Build history of the part. All positions in model axes, mm. Give positions to 0.01 mm unless a question says otherwise; leave off trailing zeros. Order: outer loops, then holes, each group sorted by start corner. A loop starts at its lowest first (then second) coordinate and runs counter-clockwise, first axis right, second up. Notation, with made-up numbers: (79.25, 54.25) - (131.25, 54.25) arc R20 cw to (131.25, 73.25) - close; hole circle Ø4 at (40.25, -10). An arc over 180 degrees is marked (long way). Answer in a Markdown table with one row per item.
```python
from build123d import *

# Parameters (mm, degrees)
F1_DEPTH = 7.5
F3_DEPTH = 25
F5_DEPTH = 25
F6_W     = 60
F6_H     = 10
F7_DEPTH = 25
F8_R     = 10


with BuildPart() as f1:
    # F0 (on Front) → F1 (new body)
    with BuildSketch(Plane.XZ):
        with BuildLine():
            Line((-64.5, -10), (-64.5, 10))
            Line((-64.5, 10), (-36.2157287525, 10))
            ThreePointArc((-36.2157287525, 10), (-94.5, 0), (-36.2157287525, -10))
            Line((-36.2157287525, -10), (-64.5, -10))
        make_face()
        with BuildLine():
            Line((-36.2157287525, 10), (-64.5, 10))
            Line((-64.5, 10), (-64.5, -10))
            Line((-64.5, -10), (-36.2157287525, -10))
            ThreePointArc((-36.2157287525, -10), (-34.9320432104, -5.0730593618), (-34.5, 0))
            ThreePointArc((-34.5, 0), (-34.9320432104, 5.0730593618), (-36.2157287525, 10))
        make_face()
        with BuildLine():
            Line((47.1794919243, 10), (-36.2157287525, 10))
            ThreePointArc((-36.2157287525, 10), (-34.9320432104, 5.0730593618), (-34.5, 0))
            ThreePointArc((-34.5, 0), (-34.9320432104, -5.0730593618), (-36.2157287525, -10))
            Line((-36.2157287525, -10), (47.1794919243, -10))
            ThreePointArc((47.1794919243, -10), (44.5, 0), (47.1794919243, 10))
        make_face()
        with BuildLine():
            ThreePointArc((84.5, 0), (69.6763809021, 19.3185165258), (47.1794919243, 10))
            Line((47.1794919243, 10), (64.5, 10))
            Line((64.5, 10), (64.5, -10))
            Line((64.5, -10), (47.1794919243, -10))
            ThreePointArc((47.1794919243, -10), (69.6763809021, -19.3185165258), (84.5, 0))
        make_face()
        with BuildLine():
            Line((64.5, 10), (47.1794919243, 10))
            ThreePointArc((47.1794919243, 10), (44.5, 0), (47.1794919243, -10))
            Line((47.1794919243, -10), (64.5, -10))
            Line((64.5, -10), (64.5, 10))
        make_face()
    extrude(amount=F1_DEPTH)

    # F2 (on face) → F3 (cut)
    with BuildSketch(Plane.XZ.offset(7.5)):
        Polygon((-52.9529946162, 20), (-76.0470053838, 20), (-87.5940107676, 0), (-76.0470053838, -20), (-52.9529946162, -20), (-41.4059892324, 0), align=None)
    extrude(amount=-F3_DEPTH, mode=Mode.SUBTRACT)

    # F4 (on face) → F5 (cut)
    with BuildSketch(Plane.XZ.offset(7.5)):
        Polygon((73.3167787844, -12.1352549156), (78.7658477444, 4.6352549156), (64.5, 15), (50.2341522556, 4.6352549156), (55.6832212156, -12.1352549156), align=None)
    extrude(amount=-F5_DEPTH, mode=Mode.SUBTRACT)

    # F6 (on face) → F7 (cut)
    with BuildSketch(Plane.XZ.offset(7.5)):
        with Locations((6.0453672857, 0)):
            Rectangle(F6_W, F6_H)
        with BuildLine():
            ThreePointArc((-23.9546327143, 5), (-28.9546327143, 0), (-23.9546327143, -5))
            Line((-23.9546327143, -5), (-23.9546327143, 5))
        make_face()
        with BuildLine():
            Line((36.0453672857, 5), (36.0453672857, -5))
            ThreePointArc((36.0453672857, -5), (41.0453672857, 0), (36.0453672857, 5))
        make_face()
    extrude(amount=-F7_DEPTH, mode=Mode.SUBTRACT)

    # F8
    f8_edges = [f1.edges().sort_by_distance(p)[0] for p in [
        (-36.215729, -3.75, -10),
        (47.179492, -3.75, 10),
        (47.179492, -3.75, -10),
        (-36.215729, -3.75, 10),
    ]]
    fillet(f8_edges, radius=F8_R)


solid = f1.part
```
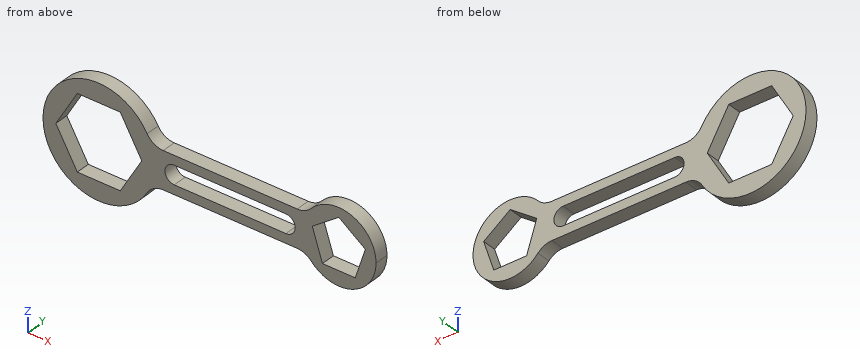
1. Drop flat-ended pins along their axis: P1, Ø1, axis at y = -2.5, z = -6, coming from the +X side; P2, Ø2, axis at x = -4, y = -2, coming from the +Z side; P3, Ø2, axis at x = 20, y = -4, coming from the -Z side. Give the stop position or say it passes through.
Check result:
| item | result |
|---|---|
| P1 | stops at x = 83.73 |
| P2 | stops at z = 10 |
| P3 | stops at z = -10 |
2. Probe line 1 (Z direction, x = -14, y = -4.5); line 2 (X direction, y = -4.5, z = 13); line 3 (X direction, y = -6, z = -8). List the from-to ranges inside material, lowest first.
Check result:
| item | result |
|---|---|
| line 1 | z = -10 to -5, 5 to 10 |
| line 2 | x = -91.54 to -80.09, -48.91 to -37, 49.28 to 61.75, 67.25 to 79.7 |
| line 3 | x = -93.41 to -82.98, -46.02 to 54.34, 74.66 to 82.83 |
3. Cut at C-C on x = 28. Write the cut outline in (y, z).
Check result:
| item | result |
|---|---|
| outline | (-7.5, -10) - (0, -10) - (0, -5) - (-7.5, -5) - close; (-7.5, 5) - (0, 5) - (0, 10) - (-7.5, 10) - close |
4. Cut at B-B on y = -3.75. Write the cut outline in (x, z), and give its area (3 significant figures).
Check result:
| item | result |
|---|---|
| outline | (-38.52, -15) arc R10 cw to (-29.86, -10) - (42.14, -10) arc R10 cw to (49.59, -13.33) arc R20 ccw (long way) to (49.59, 13.33) arc R10 cw to (42.14, 10) - (-29.86, 10) arc R10 cw to (-38.52, 15) arc R30 ccw (long way) to start; hole (-87.59, 0) - (-76.05, -20) - (-52.95, -20) - (-41.41, 0) - (-52.95, 20) - (-76.05, 20) - close; hole (-23.95, -5) - (36.05, -5) arc R5 ccw to (36.05, 5) - (-23.95, 5) arc R5 ccw to start; hole (50.23, 4.64) - (55.68, -12.14) - (73.32, -12.14) - (78.77, 4.64) - (64.5, 15) - close |
| area | 3,110 mm² |
5. Cut at A-A on x = -64.5. Write the cut outline in (y, z), and give its area (3 significant figures).
Check result:
| item | result |
|---|---|
| outline | (-7.5, -30) - (0, -30) - (0, -20) - (-7.5, -20) - close; (-7.5, 20) - (0, 20) - (0, 30) - (-7.5, 30) - close |
| area | 150 mm² |
